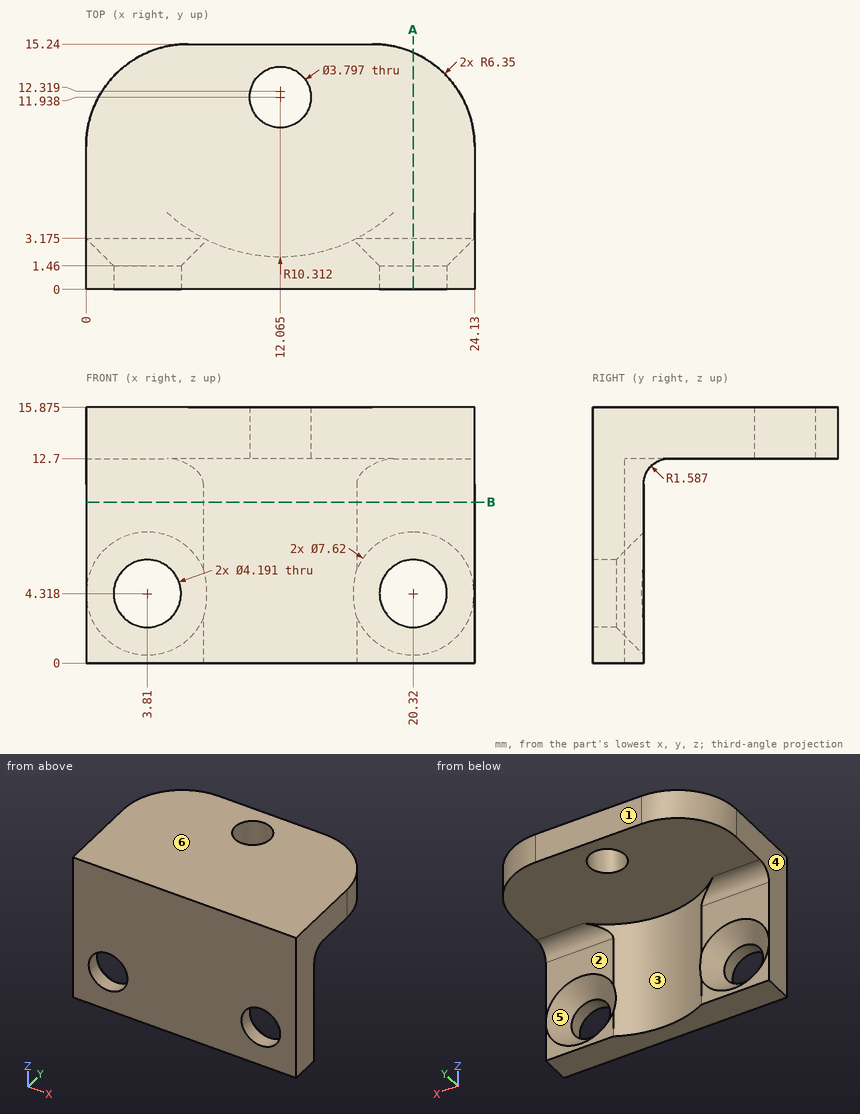
Study the drawing (mm; zero at the part's minimum x, y, z) and answer. A direction names the side the tool comes from. Give positions to 0.01 mm unless a question says otherwise; leave off trailing zeros. Loops run counter-clockwise (first coordinate to the right, second up) from the corner with the lowest first, then second, coordinate; pieces in that order, holes last. Notation, with made-up numbers: M 57,26 L 78,26 A23 ccw 78,49 Z; hole C -1.75,38 d2. An arc over 180 degrees is marked long. Answer as CSV lines item,"result".
Item 1: Which of the six approach directions +Z, -Z, +X, -X, +Y, -Y give full straight-line access (tool end or side, diameter ignored) to the marked faces 1, 2 and 3?
Values follow:
face 1,"+Z, -Z, +X, -X, +Y"
face 2,"-Z, +X, -X, +Y"
face 3,"-Z, +Y"
Item 2: The mould has two halves that part along X. Classify the marked faces 4, 5 and 6: released by +X, released by -X, zero draft, split by the parting line, or undercut.
Values follow:
face 4,"released by -X"
face 5,"undercut"
face 6,"zero draft"
Item 3: The part is cut by section B-B (z = 10). Give the vertices of the cut face in (x, y) (1 decimal).
Values follow:
outline,"M 0,0 L 24.1,0 L 24.1,3.2 L 16.8,3.2 A10.3 cw 7.3,3.2 L 0,3.2 Z"
Item 4: The part is cut by section A-A (x = 20.32). Give the vertices of the cut face in (y, z) (1 decimal).
Values follow:
outline,"M 0,0 L 3.2,0 L 3.2,0.5 L 1.5,2.2 L 0,2.2 Z; M 0,6.4 L 1.5,6.4 L 3.2,8.1 L 3.2,11.1 A1.6 cw 4.8,12.7 L 14.7,12.7 L 14.7,15.9 L 0,15.9 Z"
Item 5: Given pin 1 Ø2 at (x, z) = (3.5, 8) entering from +Y (1 decimal); pin 2 Ø2 at (x, z) = (19.5, 3) entering from +Y; pin 3 Ø2.5 at (x, y) = (12.065, 11.938) entering from +Z; pin 4 Ø1.3 at (x, z) = (5, 2.5) entering from +Y, each flat-ended and moving along its own axis, determine where each tip first touches the part or whether it passes through.
Values follow:
pin 1,"stops at y = 3.2"
pin 2,"stops at y = 1.92"
pin 3,"passes through"
pin 4,"stops at y = 2.19"
Item 6: Straight lines are drawn through the part: line 1 along Z through (x, y) = (11.75, 6.75) (1 decimal); line 2 along Y through (x, z) = (17.75, 1.25) (1 decimal); line 3 along Y through (x, z) = (7.75, 3.5). For each, find the intervals that lie inside material, in ascending order. Write a range as [from, to].
Values follow:
line 1,"z = [12.7, 15.9]"
line 2,"y = [0, 3.2]"
line 3,"y = [0, 2.95]"
